Source: CAD feature listing. Evaluate the final solid. Frame: model axes, mm. A direction names the side the tool comes from. Coordinates: 2 decimals unless noted, no trailing zeros. Loops run counter-clockwise (first coordinate to the right, second up) from the corner with the lowest first, then second, coordinate; pieces in that order, holes last. Notation, with made-up numbers: (86.25, -37.75) -> (94.25, -37.75) arc R16 ccw to (94.25, -10.75) -> close; hole circle Ø3 at (66, -3.5). An arc over 180 degrees is marked (long way). Answer as CSV lines item,"result".
from build123d import *

# Parameters (mm, degrees)
F1_R     = 4.8514
F2_DEPTH = 12.7
F4_DEPTH = 12.701


with BuildPart() as f2:
    # F1 (on Front) → F2 (new body)
    with BuildSketch(Plane.XZ):
        with BuildLine():
            ThreePointArc((-27.966589, 6), (-29.911259, 6.305105), (-31.669054, 7.1911))
            ThreePointArc((-31.669054, 7.1911), (-45.6814, 0), (-31.669054, -7.1911))
            ThreePointArc((-31.669054, -7.1911), (-29.911259, -6.305105), (-27.966589, -6))
            Line((-27.966589, -6), (27.966589, -6))
            ThreePointArc((27.966589, -6), (29.911259, -6.305105), (31.669054, -7.1911))
            ThreePointArc((31.669054, -7.1911), (45.6814, 0), (31.669054, 7.1911))
            ThreePointArc((31.669054, 7.1911), (29.911259, 6.305105), (27.966589, 6))
            Line((27.966589, 6), (-27.966589, 6))
        make_face()
        with Locations((-36.83, 0)):
            Circle(F1_R, mode=Mode.SUBTRACT)
        with Locations((36.83, 0)):
            Circle(F1_R, mode=Mode.SUBTRACT)
    extrude(amount=F2_DEPTH)

    # F3 (on Front) → F4 (cut, through all)
    with BuildSketch(Plane.XZ):
        with BuildLine():
            ThreePointArc((-24, 2), (-26, 0), (-24, -2))
            Line((-24, -2), (24, -2))
            ThreePointArc((24, -2), (26, 0), (24, 2))
            Line((24, 2), (-24, 2))
        make_face()
    extrude(amount=F4_DEPTH, mode=Mode.SUBTRACT)


solid = f2.part
(1) Cut plane C-C (y = -8). Return the cut outline in (x, z), then the cut area to 3 significant figures.
Computed values:
outline,"(-31.67, -7.19) arc R6.35 cw to (-27.97, -6) -> (27.97, -6) arc R6.35 cw to (31.67, -7.19) arc R8.85 ccw (long way) to (31.67, 7.19) arc R6.35 cw to (27.97, 6) -> (-27.97, 6) arc R6.35 cw to (-31.67, 7.19) arc R8.85 ccw (long way) to start; hole circle Ø9.7 at (-36.83, 0); hole (-24, -2) -> (24, -2) arc R2 ccw to (24, 2) -> (-24, 2) arc R2 ccw to start; hole circle Ø9.7 at (36.83, 0)"
area,"831 mm^2"
(2) Draft query along X for faces 4 (the flat face through (-1, 0, -4)), 5 (the cylindrical face through (29.9, -6.3, 6.3)), 6 (the cylindrical face through (41.457, -6.261, 1.457)). Return one class per face: released by +X, released by -X, zero draft, split by the parting line, or undercut.
Computed values:
face 4,"zero draft"
face 5,"undercut"
face 6,"undercut"
(3) Access query for faces 1 (the cylindrical face through (-26, -6, 0)), 2 (the flat face through (0, -6, 6)), 3 (the cylindrical face through (29.9, -6.3, -6.3)). Directions: +Z, -Z, +X, -X, +Y, -Y. A direction counts if a zero-diameter tool reaches every point of the face in a straight line with its end or side. Return the directions, or none.
Computed values:
face 1,"+Y, -Y"
face 2,"+Z, +Y, -Y"
face 3,"-Z, +Y, -Y"
(4) Pin query (flat end, axial travel): pin 1 Ø4 at (x, y) = (26.5, -7.5) entering from +Z; pin 2 Ø4 at (x, y) = (-5.5, -5.5) entering from -Z; pin 3 Ø4 at (y, z) = (-2, 3) entering from -X. Return the tip coordinate at first contact, or that it passes through.
Computed values:
pin 1,"z = 6.02"
pin 2,"z = -6"
pin 3,"x = -45.62"
(5) Cut plane D-D (x = 38). Return the cut outline in (y, z), then the cut area to 3 significant figures.
Computed values:
outline,"(-12.7, -8.77) -> (0, -8.77) -> (0, -4.71) -> (-12.7, -4.71) -> close; (-12.7, 4.71) -> (0, 4.71) -> (0, 8.77) -> (-12.7, 8.77) -> close"
area,"103 mm^2"
(6) Material intervals for L1, parallel to X at y = -9.5, z = -0.25; L2, parallel to Z at x = -36.83, y = -9.75; L3, parallel to X at y = -7.5, z = -3.5, sorted ascending. Write a range as [from, to].
Computed values:
L1,"[-45.68, -41.67], [-31.99, -25.98], [25.98, 31.99], [41.67, 45.68]"
L2,"[-8.85, -4.85], [4.85, 8.85]"
L3,"[-44.96, -40.19], [-33.47, 33.47], [40.19, 44.96]"
(7) Cut plane A-A (z = 0). Return the cut outline in (x, y).
Computed values:
outline,"(-45.68, -12.7) -> (-41.68, -12.7) -> (-41.68, 0) -> (-45.68, 0) -> close; (-31.98, -12.7) -> (-26, -12.7) -> (-26, 0) -> (-31.98, 0) -> close; (26, -12.7) -> (31.98, -12.7) -> (31.98, 0) -> (26, 0) -> close; (41.68, -12.7) -> (45.68, -12.7) -> (45.68, 0) -> (41.68, 0) -> close"
(8) Cut plane B-B (x = -36.83). Return the cut outline in (y, z), then the cut area to 3 significant figures.
Computed values:
outline,"(-12.7, -8.85) -> (0, -8.85) -> (0, -4.85) -> (-12.7, -4.85) -> close; (-12.7, 4.85) -> (0, 4.85) -> (0, 8.85) -> (-12.7, 8.85) -> close"
area,"102 mm^2"
